Geometry: final body of the model. Coordinates: model frame, mm. A direction names the side the tool comes from. Give positions to 0.01 mm unless a question says otherwise; leave off trailing zeros.
```python
from build123d import *

# Parameters (mm, degrees)
SKETCH004_R     = 22.270316
POCKET_DEPTH    = 45.906105
SKETCH005_R     = 15.471948
POCKET001_DEPTH = 5


with BuildPart() as part:
    # Sketch001 → Revolution (revolve)
    with BuildSketch(Plane.XZ):
        with BuildLine():
            Line((0, -6), (-40, -6))
            Line((-40, -6), (-55, -6))
            ThreePointArc((-40, 0), (-48.077747, -1.555632), (-55, -6))
            Line((-40, 0), (0, 0))
            Line((0, -6), (0, 0))
        make_face()
    revolve(axis=Axis((0, 0, 0), (0, 0, 1)))

    # Sketch003 (on Face2 of Revolution) → AdditiveLoft section 0
    with BuildSketch(Plane(origin=(0, 0, 0), x_dir=(-1, 0, 0), z_dir=(0, 0, 1))):
        Polygon((-6, 39.54744), (6, 39.54744), (6, 6), (39.54744, 6), (39.54744, -6), (6, -6), (6, -39.54744), (-6, -39.54744), (-6, -6), (-39.54744, -6), (-39.54744, 6), (-6, 6), align=None)
    # Sketch002 (on Face2 of Revolution) → AdditiveLoft section 1
    with BuildSketch(Plane(origin=(0, 0, 80), x_dir=(-1, 0, 0), z_dir=(0, 0, 1))):
        Polygon((-3, 14.696938), (3, 14.696938), (3, 3), (14.696938, 3), (14.696938, -3), (3, -3), (3, -14.696938), (-3, -14.696938), (-3, -3), (-14.696938, -3), (-14.696938, 3), (-3, 3), align=None)
    loft()

    # Sphere → Sphere (revolve)
    with BuildSketch(Plane(origin=(0, 0, 80), x_dir=(-1, 0, 0), z_dir=(0, 1, 0))):
        with BuildLine():
            ThreePointArc((0, -25), (25, 0), (0, 25))
            Line((0, 25), (0, -25))
        make_face()
    revolve(axis=Axis((0, 0, 80), (0, 0, 1)))

    # Sketch004 (on DatumPlane) → Pocket (cut, through all)
    with BuildSketch(Plane(origin=(0, -30.371881, 29.538427), x_dir=(-1, 0, 0), z_dir=(0, -0.954987, 0.296649))):
        with Locations((0, -58.80426)):
            Circle(SKETCH004_R)
    extrude(amount=POCKET_DEPTH, mode=Mode.SUBTRACT)

    # Sketch005 (on Face25 of Pocket) → Pocket001 (cut)
    with BuildSketch(Plane(origin=(0, -13.403601, 84.163578), x_dir=(1, 0, 0), z_dir=(0, -0.954987, 0.296649))):
        Circle(SKETCH005_R)
    extrude(amount=-POCKET001_DEPTH, mode=Mode.SUBTRACT)


solid = part.part
```
Q1. Material intervals for probe 1 along X at (y, z) = (-10.5, 85); probe 2 along Z at (x, y) = (-15.5, 23); probe 3 along Y at (x, z) = (0, 24), sorted ascending.
Q2. Pin query (flat end, axial travel): pin 1 Ø6 at (x, z) = (-7, 23.5) entering from +Y; pin 2 Ø2 at (x, z) = (9, 19.5) entering from -Y; pin 3 Ø10 at (x, y) = (-30.5, -36.5) entering from +Z. Return the tip coordinate at first contact, or that it passes through.
Q3. Reachability of faces 4 (the face through (-19, -19, 0)), 5 (the face through (-19, 19, 0)), 6 (the face through (19, 19, 0)) from +Z, -Z, +X, -X, +Y, -Y: full face, straight path, thin tool, end or side. Return the list, or none.
Q4. Mould query, pull axis Z, two halves, no side actions, for faces 1 (the face through (19, -19, 0)), 2 (the face through (-1, -1, -6)), 3 (the face through (7.76, -9.34, 97.25)). Classes: +Z half, -Z half, draft (parallel to the pull), parting line (faces both ways), or undercut.
Resolved:
1. probe 1: x = -22.13 to -15.38, 15.38 to 22.13
1. probe 2: z = -6 to 0
1. probe 3: y = -32.09 to 32.09
2. pin 1: stops at y = 33
2. pin 2: stops at y = -5.31
2. pin 3: stops at z = -0.15
3. face 4: -X, -Y
3. face 5: -X, +Y
3. face 6: +X, +Y
4. face 1: undercut
4. face 2: -Z half
4. face 3: +Z half
